```python
from build123d import *

# Parameters (mm, degrees)
F2_W = 8.89
F2_H = 5.08


with BuildPart() as f1:
    # F0 (on Front) → F1 (revolve)
    with BuildSketch(Plane.XZ):
        Polygon((19.05, 31.75), (0, 31.75), (0, 0), (346.71, 0), (346.71, 45.72), (341.63, 45.72), (341.63, 39.37), (322.58, 39.37), (322.58, 33.02), (309.88, 33.02), (309.88, 26.67), (284.48, 26.67), (284.48, 33.02), (278.13, 33.02), (278.13, 41.91), (259.08, 41.91), (259.08, 45.72), (252.73, 45.72), (252.73, 26.67), (100.33, 26.67), (93.98, 26.67), (93.98, 29.21), (85.09, 29.21), (85.09, 31.75), (21.59, 31.75), (21.59, 29.21), (19.05, 29.21), align=None)
    revolve(axis=Axis((173.355, 0, 0), (-1, 0, 0)))

    # F2 (on Front) → F3 (revolve)
    with BuildSketch(Plane.XZ):
        with Locations((116.205, 29.21)):
            Rectangle(F2_W, F2_H)
    revolve(axis=Axis((173.355, 0, 0), (-1, 0, 0)))


solid = f1.part
```
CAD build for the part. Positions are in the model's coordinates, mm. A direction names the side the tool comes from. Round coordinates to 2 decimals unless told otherwise and drop trailing zeros. Order: outer loops, then holes, each group sorted by start corner. A loop starts at its lowest first (then second) coordinate and runs counter-clockwise, first axis right, second up.
Q1. Slice it at B-B (x = 89.5). Write the cut outline in (y, z), and give its area (3 significant figures).
Q2. Drop flat-ended pins along their axis: pin 1 (8 mm diameter, centred on x = 85.5, z = 2.5, fed in from -Y); pin 2 (12 mm diameter, centred on x = 35.5, z = 31.5, fed in from +Y); pin 3 (3 mm diameter, centred on y = -35, z = -30.5, fed in from -X). Give the stop position or say it passes through.
Q3. Two-plate mould, pull along X, no slides. Class faces 4 (the flat face through (346.71, 1, 1)), 5 (the cylindrical face through (52.896, -30.995, -6.883)), 6 (the flat face through (21.59, -26, 14)), 7 (the cylindrical face through (89.47, 19.74, -21.53)): pulls with the +X half, pulls with the -X half, needs draft (parallel to the pull), parting line crosses it, or undercut.
Q4. Wall check: L1, parallel to X at y = -29.5, z = -27; L2, parallel to Z at x = 323.5, y = -21.5; L3, parallel to Y at x = 15, z = -10. Give the ranges that are in metal, low to high.
Q5. Which spindle directions (+Z, -Z, +X, -X, +Y, -Y) get a long thin tool onto all of the face, cutting with end or side? Do faces 1 (the cylindrical face through (344.13, 13.73, 43.61)), 2 (the cylindrical face through (116.267, -30.995, -6.883)), 3 (the cylindrical face through (297.002, 26.443, -3.472)). Say none if no direction does.
Q6. Slice it at A-A (x = 44.5). Write the cut outline in (y, z).
Results below:
1. outline: circle Ø58.42 at (0, 0)
1. area: 2,680 mm2
2. pin 1: stops at y = -31.75
2. pin 2: stops at y = 18.92
2. pin 3: stops at x = 252.73
3. face 4: pulls with the +X half
3. face 5: needs draft
3. face 6: undercut
3. face 7: undercut
4. L1: x = 252.73 to 278.13, 341.63 to 346.71
4. L2: z = -32.98 to 32.98
4. L3: y = -30.13 to 30.13
5. face 1: +X, -X
5. face 2: -X
5. face 3: none
6. outline: circle Ø63.5 at (0, 0)
